from build123d import *

# Parameters (mm, degrees)
SKETCH1_W           = 28.32
SKETCH1_H           = 25.78
SKETCH1_R           = 1.2
BOSS_EXTRUDE1_DEPTH = 3
SKETCH4_W           = 25.78
SKETCH4_H           = 28.32
SKETCH4_R           = 1.2
BOSS_EXTRUDE2_DEPTH = 4
SKETCH5_W           = 10
SKETCH5_H           = 10
CUT_EXTRUDE2_DEPTH  = 4
SKETCH8_W           = 10
SKETCH8_H           = 10
CUT_EXTRUDE3_DEPTH  = 3
BOSS_EXTRUDE3_DEPTH = 10
SKETCH3_R           = 2.9
CUT_EXTRUDE4_DEPTH  = 1.2
CHAMFER1_SIZE       = 1.5
BOSS_EXTRUDE4_DEPTH = 3
EXTRUDE_THIN1_START = -3
EXTRUDE_THIN1_DEPTH = 40
CUT_EXTRUDE5_DEPTH  = 1.7
CHAMFER2_SIZE       = 0.5
CUT_EXTRUDE6_DEPTH  = 1.2


with BuildPart() as part:
    # Sketch1 → Boss-Extrude1 (new body)
    with BuildSketch(Plane(origin=(0, 0, 0), x_dir=(1, 0, 0), z_dir=(0, 1, 0))):
        Rectangle(SKETCH1_W, SKETCH1_H)
        with Locations(Location((-10.16, 8.89, 0), (0, 0, 270))):
            Circle(SKETCH1_R, mode=Mode.SUBTRACT)
        with Locations(Location((10.16, 8.89, 0), (0, 0, 270))):
            Circle(SKETCH1_R, mode=Mode.SUBTRACT)
        with Locations(Location((10.16, -8.89, 0), (0, 0, 270))):
            Circle(SKETCH1_R, mode=Mode.SUBTRACT)
        with Locations(Location((-10.16, -8.89, 0), (0, 0, 270))):
            Circle(SKETCH1_R, mode=Mode.SUBTRACT)
    extrude(amount=BOSS_EXTRUDE1_DEPTH)

    # Sketch8 → Cut-Extrude3 (cut)
    with BuildSketch(Plane.XZ):
        with Locations((-9.16, 7.89)):
            Rectangle(SKETCH8_W, SKETCH8_H)
        with Locations((9.16, -7.89)):
            Rectangle(SKETCH8_W, SKETCH8_H)
    extrude(amount=-CUT_EXTRUDE3_DEPTH, mode=Mode.SUBTRACT)



with BuildPart() as body_2:
    # Sketch4 → Boss-Extrude2 (new body)
    with BuildSketch(Plane(origin=(0, 13, 0), x_dir=(1, 0, 0), z_dir=(0, 1, 0))):
        Rectangle(SKETCH4_W, SKETCH4_H)
        with Locations(Location((-8.89, 10.16, 0), (0, 0, 270))):
            Circle(SKETCH4_R, mode=Mode.SUBTRACT)
        with Locations(Location((8.89, 10.16, 0), (0, 0, 270))):
            Circle(SKETCH4_R, mode=Mode.SUBTRACT)
        with Locations(Location((-8.89, -10.16, 0), (0, 0, 270))):
            Circle(SKETCH4_R, mode=Mode.SUBTRACT)
        with Locations(Location((8.89, -10.16, 0), (0, 0, 270))):
            Circle(SKETCH4_R, mode=Mode.SUBTRACT)
    extrude(amount=BOSS_EXTRUDE2_DEPTH)

    # Sketch5 → Cut-Extrude2 (cut)
    with BuildSketch(Plane(origin=(0, 17, 0), x_dir=(1, 0, 0), z_dir=(0, 1, 0))):
        with Locations((-7.89, 9.16)):
            Rectangle(SKETCH5_W, SKETCH5_H)
        with Locations((7.89, -9.16)):
            Rectangle(SKETCH5_W, SKETCH5_H)
    extrude(amount=-CUT_EXTRUDE2_DEPTH, mode=Mode.SUBTRACT)


with BuildPart() as part_1:
    add(part.part)

    add(body_2.part)  # Boss-Extrude3 merges body 2
    # Sketch9 → Boss-Extrude3 (add)
    with BuildSketch(Plane.XZ.offset(-13)):
        Polygon((2.89, 4.16), (2.89, 12.89), (-4.16, 12.89), (-4.16, 2.89), (-12.89, 2.89), (-12.89, -4.16), (-2.89, -4.16), (-2.89, -12.89), (4.16, -12.89), (4.16, -2.89), (12.89, -2.89), (12.89, 4.16), align=None)
    extrude(amount=BOSS_EXTRUDE3_DEPTH)

    # Sketch3 → Cut-Extrude4 (cut)
    with BuildSketch(Plane(origin=(0, 17, 0), x_dir=(1, 0, 0), z_dir=(0, 1, 0))):
        with Locations(Location((8.89, 10.16, 0), (0, 0, 270))):
            Circle(SKETCH3_R)
        with Locations(Location((-8.89, -10.16, 0), (0, 0, 270))):
            Circle(SKETCH3_R)
    extrude(amount=-CUT_EXTRUDE4_DEPTH, mode=Mode.SUBTRACT)

    # Chamfer1
    # the kernel refuses this chamfer: 1.5 mm, written as the material it adds along each edge
    with BuildSketch(Plane(origin=(-2.89, 13, -12.89), x_dir=(0, -0.9996219169112968, 0.027495876610585616), z_dir=(1, 0, 0))) as chamfer1_piece_1_section:
        Polygon((CHAMFER1_SIZE * 0.999621916911, CHAMFER1_SIZE * 0.0274958766106), (-CHAMFER1_SIZE * 0.0274958766106, CHAMFER1_SIZE * 0.999621916911), (0, 0), align=None)
    chamfer1_piece_1 = extrude(amount=7.05, mode=Mode.PRIVATE)
    chamfer1_piece_1 = split(chamfer1_piece_1, bisect_by=Plane(origin=(0.635, 12.489006397, -14.16), z_dir=(0, 0, 1)), keep=Keep.TOP, mode=Mode.PRIVATE)
    add(chamfer1_piece_1)
    with BuildSketch(Plane(origin=(2.89, 13, 12.89), x_dir=(0, -0.9996219169112965, -0.02749587661058676), z_dir=(-1, 0, 0))) as chamfer1_piece_2_section:
        Polygon((CHAMFER1_SIZE * 0.999621916911, CHAMFER1_SIZE * 0.0274958766106), (-CHAMFER1_SIZE * 0.0274958766106, CHAMFER1_SIZE * 0.999621916911), (0, 0), align=None)
    chamfer1_piece_2 = extrude(amount=7.05, mode=Mode.PRIVATE)
    chamfer1_piece_2 = split(chamfer1_piece_2, bisect_by=Plane(origin=(-0.635, 12.489006397, 14.16), z_dir=(0, 0, -1)), keep=Keep.TOP, mode=Mode.PRIVATE)
    add(chamfer1_piece_2)
    with BuildSketch(Plane(origin=(12.89, 3, -2.89), x_dir=(0.9996219169112965, -0.027495876610587625, 0), z_dir=(0, 0, 1))) as chamfer1_piece_3_section:
        Polygon((CHAMFER1_SIZE * 0.999621916911, CHAMFER1_SIZE * 0.0274958766106), (-CHAMFER1_SIZE * 0.0274958766106, CHAMFER1_SIZE * 0.999621916911), (0, 0), align=None)
    chamfer1_piece_3 = extrude(amount=7.05, mode=Mode.PRIVATE)
    chamfer1_piece_3 = split(chamfer1_piece_3, bisect_by=Plane(origin=(14.16, 3.510993603, 0.635), z_dir=(-1, 0, 0)), keep=Keep.TOP, mode=Mode.PRIVATE)
    add(chamfer1_piece_3)
    with BuildSketch(Plane(origin=(-12.89, 3, 2.89), x_dir=(-0.9996219169112965, -0.027495876610587625, 0), z_dir=(0, 0, -1))) as chamfer1_piece_4_section:
        Polygon((CHAMFER1_SIZE * 0.999621916911, CHAMFER1_SIZE * 0.0274958766106), (-CHAMFER1_SIZE * 0.0274958766106, CHAMFER1_SIZE * 0.999621916911), (0, 0), align=None)
    chamfer1_piece_4 = extrude(amount=7.05, mode=Mode.PRIVATE)
    chamfer1_piece_4 = split(chamfer1_piece_4, bisect_by=Plane(origin=(-14.16, 3.510993603, -0.635), z_dir=(1, 0, 0)), keep=Keep.TOP, mode=Mode.PRIVATE)
    add(chamfer1_piece_4)

    # Sketch10 → Boss-Extrude4 (add)
    with BuildSketch(Plane(origin=(0, 3, 0), x_dir=(1, 0, 0), z_dir=(0, 1, 0))):
        Polygon((-28.302135624, 12.89), (-14.16, -2.89), (-14.16, 12.89), (4.16, 12.89), (-14.16, 27.032135624), (-28.302135624, 27.032135624), align=None)
    extrude(amount=-BOSS_EXTRUDE4_DEPTH)

    # Sketch11 → Extrude-Thin1 (add)
    with BuildSketch(Plane(origin=(0, 3, 0), x_dir=(1, 0, 0), z_dir=(0, 1, 0)).offset(EXTRUDE_THIN1_START)):
        Polygon((-28.302135624, -14.16), (-28.302135624, 27.032135624), (0, 27.032135624), (0, 25.032135624), (-26.302135624, 25.032135624), (-26.302135624, -14.16), align=None)
    extrude(amount=EXTRUDE_THIN1_DEPTH)

    # Sketch12 → Cut-Extrude5 (cut)
    with BuildSketch(Plane.XZ.offset(-13)):
        Polygon((-10.076454803, 12.215), (-11.262909606, 10.16), (-10.076454803, 8.105), (-7.703545197, 8.105), (-6.517090394, 10.16), (-7.703545197, 12.215), align=None)
        Polygon((10.076454803, -12.215), (11.262909606, -10.16), (10.076454803, -8.105), (7.703545197, -8.105), (6.517090394, -10.16), (7.703545197, -12.215), align=None)
    extrude(amount=-CUT_EXTRUDE5_DEPTH, mode=Mode.SUBTRACT)

    # Chamfer2
    chamfer2_edges = [part_1.edges().sort_by_distance(p)[0] for p in [
        (-8.89, 13, 12.215),
        (-10.669682205, 13, 11.1875),
        (-10.669682205, 13, 9.1325),
        (-8.89, 13, 8.105),
        (-7.110317795, 13, 9.1325),
        (-7.110317795, 13, 11.1875),
        (8.89, 13, -12.215),
        (10.669682205, 13, -11.1875),
        (10.669682205, 13, -9.1325),
        (8.89, 13, -8.105),
        (7.110317795, 13, -9.1325),
        (7.110317795, 13, -11.1875),
    ]]
    chamfer(chamfer2_edges, length=CHAMFER2_SIZE)

    # Sketch13 → Cut-Extrude6 (cut)
    with BuildSketch(Plane(origin=(0, 17, 0), x_dir=(1, 0, 0), z_dir=(0, 1, 0))):
        with BuildLine():
            Line((-9.89, 4.16), (-9.89, -7.437868482))
            ThreePointArc((-9.89, -7.437868482), (-8.89, -7.26), (-7.89, -7.437868482))
            Line((-7.89, -7.437868482), (-7.89, 4.16))
            Line((-7.89, 4.16), (-9.89, 4.16))
        make_face()
        with BuildLine():
            ThreePointArc((9.89, 7.437868482), (8.89, 7.26), (7.89, 7.437868482))
            Line((7.89, 7.437868482), (7.89, -4.16))
            Line((7.89, -4.16), (9.89, -4.16))
            Line((9.89, -4.16), (9.89, 7.437868482))
        make_face()
    extrude(amount=-CUT_EXTRUDE6_DEPTH, mode=Mode.SUBTRACT)


solid = part_1.part
Geometry: final body of the model. Coordinates: model frame, mm. A direction names the side the tool comes from. Give positions to 0.01 mm unless a question says otherwise; leave off trailing zeros. Order: outer loops, then holes, each group sorted by start corner. A loop starts at its lowest first (then second) coordinate and runs counter-clockwise, first axis right, second up. Notation, with made-up numbers: (-7, 19) -> (8, 19) arc R16 ccw to (8, 34) -> close; hole circle Ø8 at (21.25, 4.25). An arc over 180 degrees is marked (long way). Write each question's results on one line, items separated by ' | '.
1) Cut plane D-D (x = 2). Output: boundary loops of the cut face in (y, z).
Geometry says:
outline: (0, -14.56) -> (3, -14.56) -> (3, -12.89) -> (11.5, -12.89) -> (12.77, -14.16) -> (17, -14.16) -> (17, 14.16) -> (12.77, 14.16) -> (11.5, 12.89) -> (0, 12.89) -> close
2) Draft query along X for faces 6 (the face through (-9, 14, 12.215)), 7 (the face through (-27, 40, -13)), 8 (the face through (-3.594, 1.521, -18.876)), 9 (the face through (7.119, 14.092, -9.118)). Return one class per face: released by +X, released by -X, zero draft, split by the parting line, or undercut.
Geometry says:
face 6: undercut | face 7: zero draft | face 8: released by +X | face 9: undercut
3) Cut plane C-C (y = 29). Output: boundary loops of the cut face in (x, z), and give its area (3 significant figures).
Geometry says:
outline: (-28.3, -27.03) -> (0, -27.03) -> (0, -25.03) -> (-26.3, -25.03) -> (-26.3, 14.16) -> (-28.3, 14.16) -> close | area: 135 mm²
4) Line query: line 1 along X through (y, z) = (15.4, -10.16); line 2 along X through (y, z) = (16.15, 10.16); line 3 along Z through (x, y) = (8.89, 15.4). Output: solid intervals per line, ascending.
Geometry says:
line 1: x = -28.3 to -26.3, -2.89 to 7.69, 10.09 to 12.89 | line 2: x = -28.3 to -26.3, -12.89 to -11.79, -5.99 to 2.89 | line 3: z = -14.16 to -11.36, -8.96 to 4.16
5) Cut plane A-A (z = 3.5). Output: boundary loops of the cut face in (x, y), and give its area (3 significant figures).
Geometry says:
outline: (-28.3, 0) -> (-26.3, 0) -> (-26.3, 40) -> (-28.3, 40) -> close; (-12.89, 13) -> (-4.16, 13) -> (-4.16, 0) -> (14.16, 0) -> (14.16, 3.23) -> (12.89, 4.5) -> (12.89, 17) -> (9.89, 17) -> (9.89, 15.8) -> (7.89, 15.8) -> (7.89, 17) -> (-7.89, 17) -> (-7.89, 15.8) -> (-9.89, 15.8) -> (-9.89, 17) -> (-12.89, 17) -> close | area: 405 mm²
6) First-contact query: pin 1 Ø7 at (x, z) = (8.5, -7) entering from -Y; pin 2 Ø4 at (x, z) = (-8.89, 10.16) entering from -Y; pin 3 Ø4.5 at (x, z) = (-8.89, 10.16) entering from +Y. Flat tips, straight axial feed; report the tip coordinate or a pass-through.
Geometry says:
pin 1: stops at y = 13 | pin 2: stops at y = 14.7 | pin 3: stops at y = 15.8
7) Set-up query: faces 1 (the face through (4.16, 7, -8)), 2 (the face through (9.89, 16, -2)), 3 (the face through (-6.887, 13.254, 11.293)), 4 (the face through (-9, 13, 7)), 5 (the face through (0.59, 12.13, -13.52)). Return all of +Z, -Z, +X, -X, +Y, -Y with unobstructed straight access to the full face (end or side cutting, diameter ignored); none if empty.
Geometry says:
face 1: -Z, +X, -Y | face 2: +Z, +Y | face 3: -Y | face 4: +Z, -Y | face 5: +X
8) Cut plane B-B (y = 6). Output: boundary loops of the cut face in (x, z).
Geometry says:
outline: (-28.3, -27.03) -> (0, -27.03) -> (0, -25.03) -> (-26.3, -25.03) -> (-26.3, 14.16) -> (-28.3, 14.16) -> close; (-12.89, -4.16) -> (-2.89, -4.16) -> (-2.89, -12.89) -> (4.16, -12.89) -> (4.16, -2.89) -> (12.89, -2.89) -> (12.89, 4.16) -> (2.89, 4.16) -> (2.89, 12.89) -> (-4.16, 12.89) -> (-4.16, 2.89) -> (-12.89, 2.89) -> close
